Source: CAD feature listing. Evaluate the final solid. Frame: model axes, mm. Face numbers are marked on the shaded views. A direction names the side the tool comes from. Round coordinates to 2 decimals unless told otherwise and drop trailing zeros. Write each loop counter-clockwise with the first axis right and the second up, starting at its lowest first coordinate (ties: lowest second). Pieces come first, ordered by that corner, then holes. Notation, with made-up numbers: M 31,-28.75 L 42,-28.75 A15 ccw 42,-13.75 Z; hole C 21,36.25 d2. An arc over 180 degrees is marked long. Put each result on its own line as item: value. Start each with the question number.
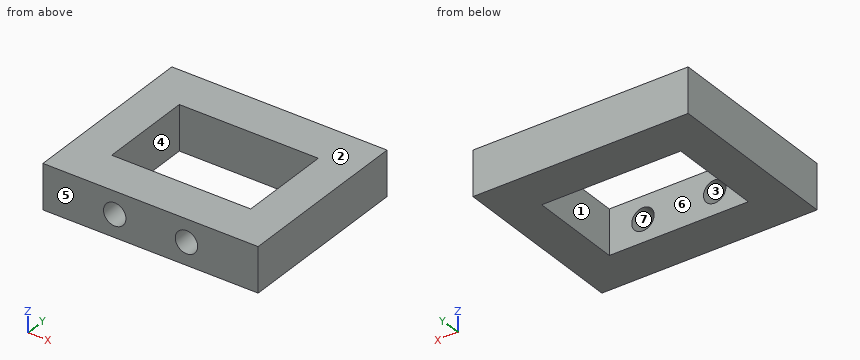
```python
from build123d import *

# Parameters (mm, degrees)
SKETCH_1_W          = 24
SKETCH_1_H          = 20
EXTRUDE_1_DEPTH     = 2.5
SKETCH_2_W          = 15.5
SKETCH_2_H          = 10.5
CUT_EXTRUDE_1_DEPTH = 6
CUT_EXTRUDE_2_REACH = 22
SKETCH_4_R          = 1.25


with BuildPart() as part:
    # 草圖1 → 填料-伸長1 (new body, symmetric)
    with BuildSketch(Plane.XY):
        Rectangle(SKETCH_1_W, SKETCH_1_H)
    extrude(amount=EXTRUDE_1_DEPTH, both=True)

    # 草圖2 → 除料-伸長1 (cut, through all)
    with BuildSketch(Plane.XY.offset(2.5)):
        Rectangle(SKETCH_2_W, SKETCH_2_H)
    extrude(amount=-CUT_EXTRUDE_1_DEPTH, mode=Mode.SUBTRACT)

    # 草圖4 → 除料-伸長2 (cut, up to next)
    with BuildSketch(Plane.XZ.offset(10), mode=Mode.PRIVATE) as cut_extrude_2_sk1:
        with Locations((-4, 0)):
            Circle(SKETCH_4_R)
    cut_extrude_2_tool1 = extrude(cut_extrude_2_sk1.sketch, amount=-CUT_EXTRUDE_2_REACH, mode=Mode.PRIVATE) & part.part
    add(cut_extrude_2_tool1.solids().sort_by_distance((-4, -10, 0))[0], mode=Mode.SUBTRACT)
    # 草圖4 → 除料-伸長2 (cut, up to next)
    with BuildSketch(Plane.XZ.offset(10), mode=Mode.PRIVATE) as cut_extrude_2_sk2:
        with Locations((4, 0)):
            Circle(SKETCH_4_R)
    cut_extrude_2_tool2 = extrude(cut_extrude_2_sk2.sketch, amount=-CUT_EXTRUDE_2_REACH, mode=Mode.PRIVATE) & part.part
    add(cut_extrude_2_tool2.solids().sort_by_distance((4, -10, 0))[0], mode=Mode.SUBTRACT)


solid = part.part
```
(1) Ray query, line 1 along Y through (x, z) = (0.25, 1.95); line 2 along X through (y, z) = (-2.5, 0.5); line 3 along Z through (x, y) = (4, -8.35). Return the intervals inside material, ascending.
(2) Contact query for a flat-ended pin moving along its axis: P1, Ø12, axis at x = -4.5, y = 0.5, coming from the +Z side. Output: stop coordinate, or through.
(3) Pull-direction query (Y, two-part tool) for the marked faces 4, 5, 6 and 7; classes: +Y half, -Y half, draft (parallel to the pull), parting line (faces both ways), or undercut.
(4) Section query A-A (x = -4). Return loops of the section in (y, z), and give its area (3 significant figures).
(5) Section query D-D (z = 2.15). Return loops of the section in (x, y).
(6) Access query for the marked faces 1, 2 and 3. Directions: +Z, -Z, +X, -X, +Y, -Y. A direction counts if a zero-diameter tool reaches every point of the face in a straight line with its end or side. Return the directions, or none.
(7) Section query C-C (z = 0). Return loops of the section in (x, y), and give its area (4 significant figures).
(8) Section query B-B (y = 0). Return loops of the section in (x, z).
Entries:
1. line 1: -10 to -5.25, 5.25 to 10
1. line 2: -12 to -7.75, 7.75 to 12
1. line 3: -2.5 to -1.25, 1.25 to 2.5
2. P1: z = 2.5
3. face 4: undercut
3. face 5: -Y half
3. face 6: undercut
3. face 7: draft
4. outline: M -10,-2.5 L -5.25,-2.5 L -5.25,-1.25 L -10,-1.25 Z; M -10,1.25 L -5.25,1.25 L -5.25,2.5 L -10,2.5 Z; M 5.25,-2.5 L 10,-2.5 L 10,2.5 L 5.25,2.5 Z
4. area: 35.6 mm2
5. outline: M -12,-10 L 12,-10 L 12,10 L -12,10 Z; hole M -7.75,-5.25 L 7.75,-5.25 L 7.75,5.25 L -7.75,5.25 Z
6. face 1: +Z, -Z
6. face 2: +Z, +X, -X, +Y, -Y
6. face 3: -Y
7. outline: M -12,-10 L -5.25,-10 L -5.25,-5.25 L -7.75,-5.25 L -7.75,5.25 L 7.75,5.25 L 7.75,-5.25 L 5.25,-5.25 L 5.25,-10 L 12,-10 L 12,10 L -12,10 Z; M -2.75,-10 L 2.75,-10 L 2.75,-5.25 L -2.75,-5.25 Z
7. area: 293.5 mm2
8. outline: M -12,-2.5 L -7.75,-2.5 L -7.75,2.5 L -12,2.5 Z; M 7.75,-2.5 L 12,-2.5 L 12,2.5 L 7.75,2.5 Z
